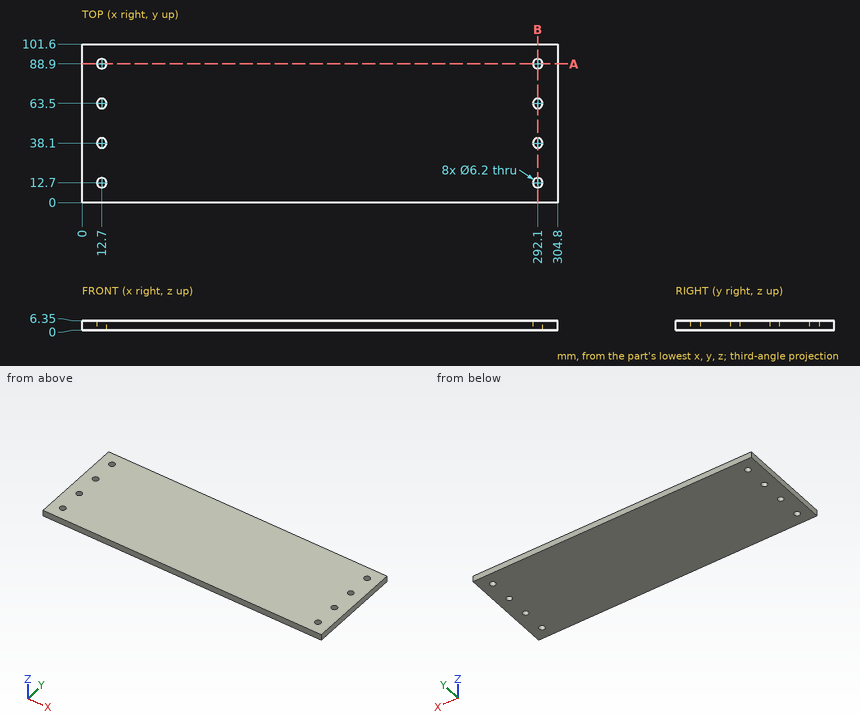
Can you work these out from the drawing? Everything is in mm from the part's minimum corner. Round coordinates to 2 decimals unless told otherwise and drop trailing zeros. Write each loop counter-clockwise with the first axis right and the second up, starting at its lowest first coordinate (ties: lowest second). Pieces come first, ordered by that corner, then holes. Notation, with made-up numbers: (-13.5, 79) - (25.5, 79) arc R20 cw to (25.5, 104) - close; hole circle Ø10 at (27.25, 13). An arc over 180 degrees is marked (long way). Put each result on its own line as item: value. Start each with the question number.
(1) Will this pin go through, and if not, where does the flat tip stop? pin 1 (5.5 mm diameter, centred on x = 292.1, y = 63.5, fed in from -Z).
(2) I want a section at A-A, the plane y = 88.9. Please give me the cut outline in (x, z), plus the area to 3 significant figures.
(3) I need wall thicknesses on probe 1 along Y at (x, z) = (292.1, 4.25); probe 2 along X at (y, z) = (88.5, 4.5). Which ranges of each line are inside material? Lowest first, please.
(4) I want a section at B-B, the plane x = 292.1. Please give me the cut outline in (y, z), plus the area to 3 significant figures.
Here are the results:
1. pin 1: passes through
2. outline: (0, 0) - (9.6, 0) - (9.6, 6.35) - (0, 6.35) - close; (15.8, 0) - (289, 0) - (289, 6.35) - (15.8, 6.35) - close; (295.2, 0) - (304.8, 0) - (304.8, 6.35) - (295.2, 6.35) - close
2. area: 1,860 mm^2
3. probe 1: y = 0 to 9.6, 15.8 to 35, 41.2 to 60.4, 66.6 to 85.8, 92 to 101.6
3. probe 2: x = 0 to 9.63, 15.77 to 289.03, 295.17 to 304.8
4. outline: (0, 0) - (9.6, 0) - (9.6, 6.35) - (0, 6.35) - close; (15.8, 0) - (35, 0) - (35, 6.35) - (15.8, 6.35) - close; (41.2, 0) - (60.4, 0) - (60.4, 6.35) - (41.2, 6.35) - close; (66.6, 0) - (85.8, 0) - (85.8, 6.35) - (66.6, 6.35) - close; (92, 0) - (101.6, 0) - (101.6, 6.35) - (92, 6.35) - close
4. area: 488 mm^2
